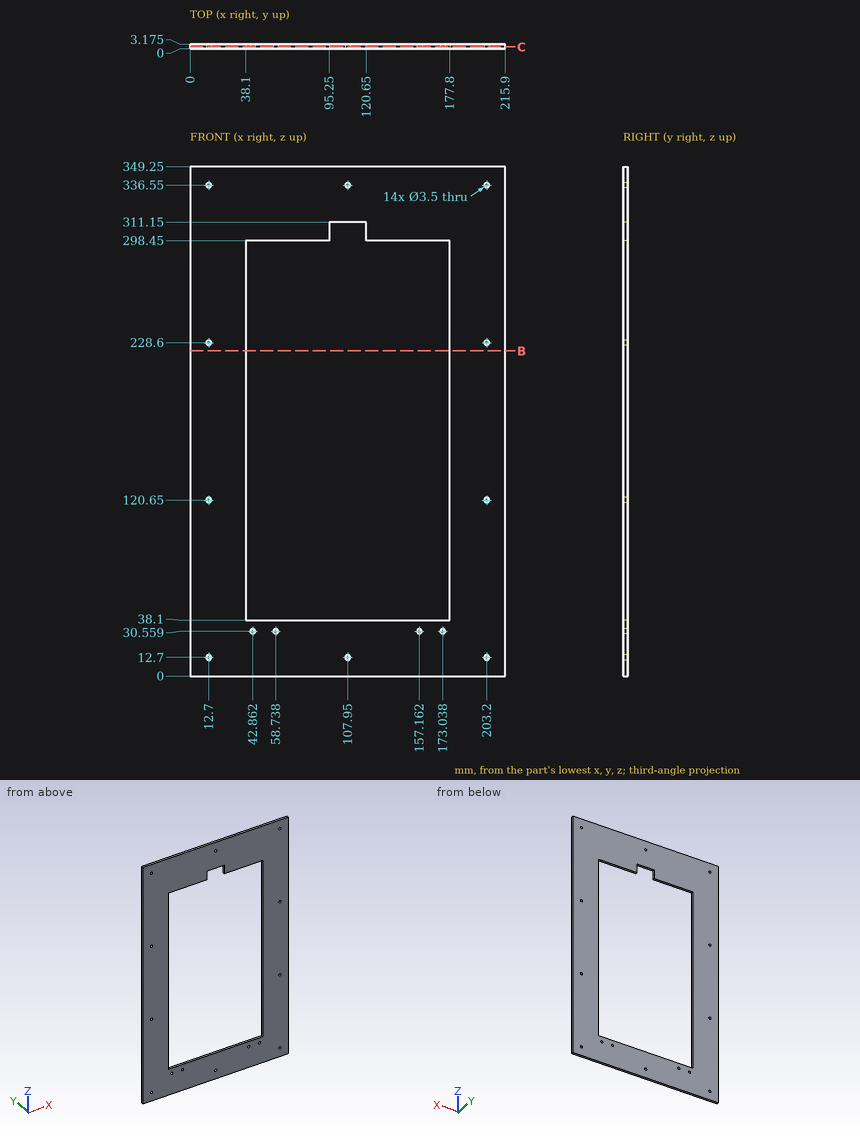
Can you work these out from the drawing? Everything is in mm from the part's minimum corner. Give positions to 0.01 mm unless a question says otherwise; leave off trailing zeros. Write each loop counter-clockwise with the first axis right and the second up, starting at its lowest first coordinate (ties: lowest second). Pieces come first, ordered by that corner, then holes. Notation, with made-up numbers: (-1, -18) -> (52, -18) arc R17 ccw to (52, -5) -> close; hole circle Ø10 at (50.5, 45). An arc over 180 degrees is marked (long way). Write each question's results on one line, items separated by ' | '. Start each with the question number.
Q1. Suppose I cut it at B-B, the plane z = 223. List the corners of the cut face in (x, y) for me (1 decimal).
Q2. Suppose I cut it at C-C, the plane y = 1.2. State how many separate pieces and enclosed holes the cut face has, and give its area (3 significant figures).
Q3. I need wall thicknesses on probe 1 along X at (y, z) = (2.05, 120.65); probe 2 along Z at (x, y) = (107.95, 0.8); probe 3 along X at (y, z) = (0.7, 336.55). Which ranges of each line are inside material? Lowest first, please.
Q4. I'm going to push flat-ended pins straight in: pin 1 Ø5.5 at (x, z) = (107.95, 12.7) entering from -Y; pin 2 Ø3 at (x, z) = (173.04, 30.56) entering from +Y. Where does each tip first touch, or does it pass through?
Outcome:
1) outline: (0, 0) -> (38.1, 0) -> (38.1, 3.2) -> (0, 3.2) -> close; (177.8, 0) -> (215.9, 0) -> (215.9, 3.2) -> (177.8, 3.2) -> close
2) separate pieces: 1 | enclosed holes: 15 | area: 38,600 mm2
3) probe 1: 0 to 10.95, 14.45 to 38.1, 177.8 to 201.45, 204.95 to 215.9 | probe 2: 0 to 10.95, 14.45 to 38.1, 311.15 to 334.8, 338.3 to 349.25 | probe 3: 0 to 10.95, 14.45 to 106.2, 109.7 to 201.45, 204.95 to 215.9
4) pin 1: y = 0 | pin 2: through
